Source: CAD feature listing. Evaluate the final solid. Frame: model axes, mm. Round coordinates to 2 decimals unless told otherwise and drop trailing zeros. Write each loop counter-clockwise with the first axis right and the second up, starting at its lowest first coordinate (ties: lowest second). Pieces come first, ordered by that corner, then holes. Notation, with made-up numbers: M 3.25,58.5 L 22.25,58.5 A19 cw 22.25,70.5 Z; hole C -28,1.25 d7. An arc over 180 degrees is marked long. Use a Markdown table: item, result.
```python
from build123d import *

# Parameters (mm, degrees)
SKETCH_1_R          = 90
EXTRUDE_1_DEPTH     = 12.6
CUT_EXTRUDE_2_DEPTH = 32
SKETCH_12_R         = 90.5
SKETCH_12_R_2       = 74
CUT_EXTRUDE_3_DEPTH = 4.5


with BuildPart() as part:
    # Эскиз1 → Вытянуть1 (new body)
    with BuildSketch(Plane(origin=(0, 0, 0), x_dir=(1, 0, 0), z_dir=(0, 1, 0))):
        with Locations(Location((0, 0, 0), (0, 0, 270))):
            Circle(SKETCH_1_R)
    extrude(amount=EXTRUDE_1_DEPTH)

    # Эскиз3 → Вырез-Вытянуть2 (cut)
    with BuildSketch(Plane.XZ):
        with BuildLine():
            Line((-2.741099481, 6.440991666), (-2.981761783, 8.569223808))
            Line((-2.981761783, 8.569223808), (0.992906346, 9.018682664))
            Line((0.992906346, 9.018682664), (1.233568648, 6.890450522))
            ThreePointArc((1.233568648, 6.890450522), (0.786552998, -6.955669226), (-2.741099481, 6.440991666))
        make_face()
    extrude(amount=-CUT_EXTRUDE_2_DEPTH, mode=Mode.SUBTRACT)

    # Эскиз4 → Вырез-Повернуть1 (revolve, cut)
    with BuildSketch(Plane.XY, mode=Mode.PRIVATE) as cut_revolve_1_sk:
        Polygon((68.863884992, 5.478404134), (72.400551948, 5.478404134), (77.896748421, -0.267847705), (63.367688519, -0.267847705), align=None)
    revolve(cut_revolve_1_sk.sketch.rotate(Axis((0, 80, 0), (0, 1, 0)), 270), axis=Axis((0, 80, 0), (0, 1, 0)), mode=Mode.SUBTRACT)

    # Эскиз7 → Вырез-Повернуть2 (revolve, cut)
    with BuildSketch(Plane.XY, mode=Mode.PRIVATE) as cut_revolve_2_sk:
        Polygon((85.06284255, 5.700411661), (87.617091847, 9.423063388), (81.248665283, 9.423063388), (83.802914581, 5.700411661), align=None)
    revolve(cut_revolve_2_sk.sketch.rotate(Axis((0, 0, 0), (0, 1, 0)), 90), axis=Axis((0, 0, 0), (0, 1, 0)), mode=Mode.SUBTRACT)

    # Эскиз12 → Вытянуть3 (cut)
    with BuildSketch(Plane(origin=(0, 12.6, 0), x_dir=(1, 0, 0), z_dir=(0, 1, 0))):
        Circle(SKETCH_12_R)
        with Locations(Location((0, 0, 0), (0, 0, 270))):
            Circle(SKETCH_12_R_2, mode=Mode.SUBTRACT)
    extrude(amount=-CUT_EXTRUDE_3_DEPTH, mode=Mode.SUBTRACT)


solid = part.part
```
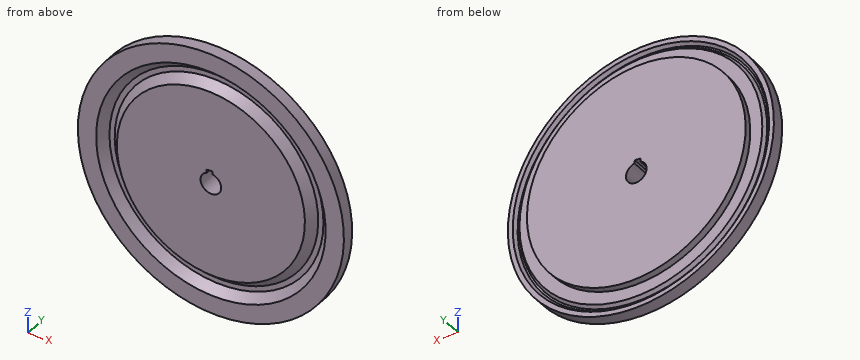
Q1. Section A-A on z = 0. Return loops of the section in (x, y), plus the area to 3 significant figures.
Results are:
| item | result |
|---|---|
| outline | M -90,0 L -77.64,0 L -72.4,5.48 L -68.86,5.48 L -63.62,0 L -7,0 L -7,12.6 L -74,12.6 L -74,8.1 L -82.16,8.1 L -83.8,5.7 L -85.06,5.7 L -86.71,8.1 L -90,8.1 Z; M 7,0 L 63.62,0 L 68.86,5.48 L 72.4,5.48 L 77.64,0 L 90,0 L 90,8.1 L 86.71,8.1 L 85.06,5.7 L 83.8,5.7 L 82.16,8.1 L 74,8.1 L 74,12.6 L 7,12.6 Z |
| area | 1,840 mm^2 |
Q2. Section B-B on y = 3. Return loops of the section in (x, z).
Results are:
| item | result |
|---|---|
| outline | C 0,0 d180; C 0,0 d132.99; hole C 0,0 d149.54; hole M -2.98,8.57 L -2.74,6.44 A7 ccw long 1.23,6.89 L 0.99,9.02 Z |
Q3. First-contact query: pin 1 Ø5 at (y, z) = (7, 31) entering from +X; pin 2 Ø12.5 at (x, z) = (0, 0) entering from +Y; pin 3 Ø4 at (x, y) = (71, 6.5) entering from -Z; pin 4 Ø1.5 at (x, z) = (-61.5, 62.5) entering from -Y. Flat tips, straight axial feed; report the tip coordinate or a pass-through.
Results are:
| item | result |
|---|---|
| pin 1 | x = 85.37 |
| pin 2 | through |
| pin 3 | z = -57.78 |
| pin 4 | y = 0 |
Q4. Line query: L1, parallel to X at y = 8, z = 31.5; L2, parallel to Z at x = 4.5, y = 6; L3, parallel to X at y = 5.25, z = 0. Output: solid intervals per line, ascending.
Results are:
| item | result |
|---|---|
| L1 | -84.31 to -80.71, -75.95 to 75.95, 80.71 to 84.31 |
| L2 | -89.89 to -85.15, -83.48 to -5.36, 5.36 to 83.48, 85.15 to 89.89 |
| L3 | -90 to -72.62, -68.65 to -7, 7 to 68.65, 72.62 to 90 |
